Study the drawing (mm; zero at the part's minimum x, y, z) and answer. A direction names the side the tool comes from. Round coordinates to 2 decimals unless told otherwise and drop trailing zeros. Loops run counter-clockwise (first coordinate to the right, second up) from the corner with the lowest first, then second, coordinate; pieces in that order, holes last. Notation, with made-up numbers: (16, 9) - (72, 9) arc R20 ccw to (72, 36) - close; hole circle Ø10 at (23.25, 67.5). An arc over 180 degrees is marked (long way). Use CSV: the item, a comma, the result in double quotes. Start each with the question number.
1. Find section C-C (y = 16.5). Give the vertices of the cut face in (x, z), and give its area (3 significant figures).
2. Find section B-B (x = 5). Give the vertices of the cut face in (y, z), and give its area (3 significant figures).
3. Given pin 1 Ø4 at (x, z) = (17.73, 4) entering from -Y; pin 2 Ø2.5 at (x, z) = (17.73, 11.5) entering from -Y; pin 3 Ø3 at (y, z) = (18.5, 8.5) entering from +X; pin 4 Ø2 at (y, z) = (22, 2.5) entering from -X, each flat-ended and moving along its own axis, determine where each tip first touches the part or whether it passes through.
4. Find section A-A (y = 5). Give the vertices of the cut face in (x, z).
5. Determine the mould class of the marked faces 5, 6, 7 and 8 for opening direction X: +X half, -X half, draft (parallel to the pull), parting line (faces both ways), or undercut.
6. A tool of negligible diameter and unlimited length cuts with its end or side. For the marked faces 1, 2, 3 and 4, from which of +Z, -Z, +X, -X, +Y, -Y can it reach the whole face along a straight path? Write none if from no direction.
7. Consider line 1 along Y through (x, z) = (5, 4.75); line 2 along X through (y, z) = (32, 12.25) (1 decimal); line 3 along Y through (x, z) = (32.5, 6.25). Determine where each line is inside the solid, lowest interval first.
8. Find section D-D (z = 12.5). State how many separate pieces and enclosed holes the cut face has, and give its area (3 significant figures).
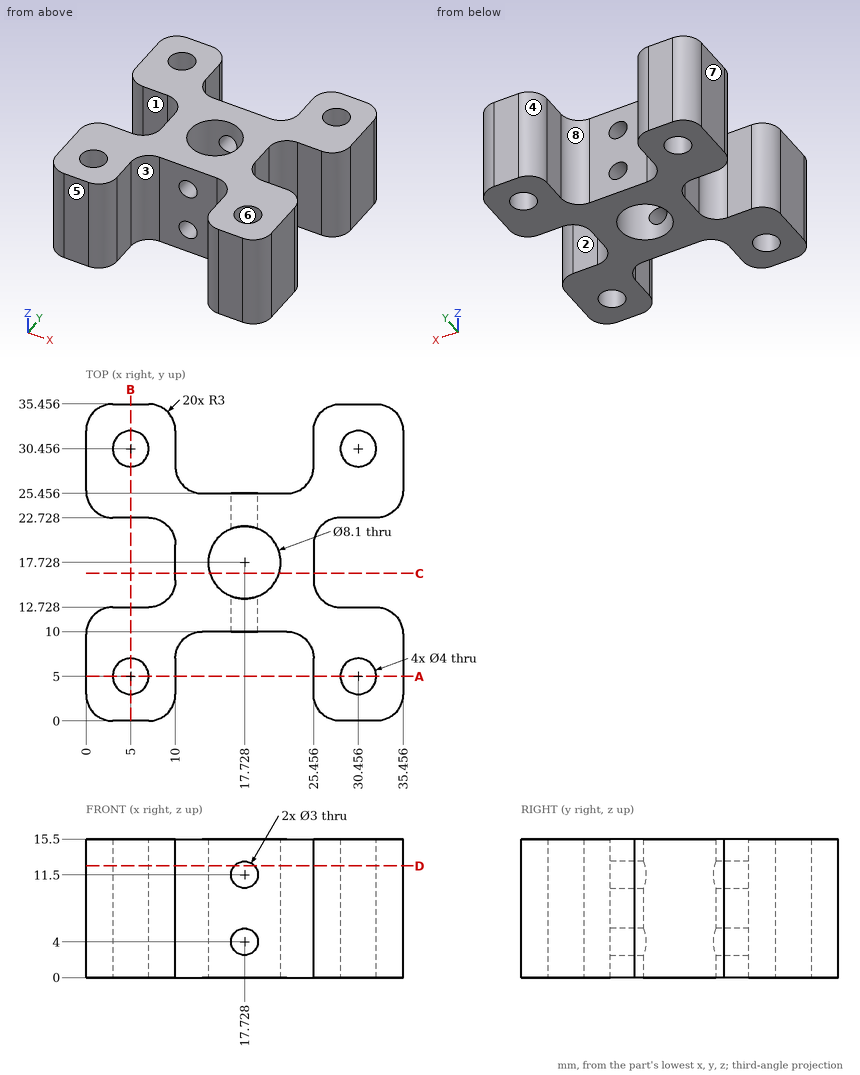
Filled sheet:
1,outline,"(10, 0) - (13.87, 0) - (13.87, 15.5) - (10, 15.5) - close; (21.59, 0) - (25.46, 0) - (25.46, 15.5) - (21.59, 15.5) - close"
1,area,"120 mm²"
2,outline,"(0, 0) - (3, 0) - (3, 15.5) - (0, 15.5) - close; (7, 0) - (12.73, 0) - (12.73, 15.5) - (7, 15.5) - close; (22.73, 0) - (28.46, 0) - (28.46, 15.5) - (22.73, 15.5) - close; (32.46, 0) - (35.46, 0) - (35.46, 15.5) - (32.46, 15.5) - close"
2,area,"271 mm²"
3,pin 1,"stops at y = 10"
3,pin 2,"passes through"
3,pin 3,"stops at x = 25.47"
3,pin 4,"stops at x = 1.75"
4,outline,"(0, 0) - (3, 0) - (3, 15.5) - (0, 15.5) - close; (7, 0) - (10, 0) - (10, 15.5) - (7, 15.5) - close; (25.46, 0) - (28.46, 0) - (28.46, 15.5) - (25.46, 15.5) - close; (32.46, 0) - (35.46, 0) - (35.46, 15.5) - (32.46, 15.5) - close"
5,face 5,"draft"
5,face 6,"undercut"
5,face 7,"-X half"
5,face 8,"undercut"
6,face 1,"+Z, -Z, -X"
6,face 2,"+Z, -Z, +X"
6,face 3,"+Z, -Z, -Y"
6,face 4,"+Z, -Z, +Y"
7,line 1,"y = 0 to 3, 7 to 12.73, 22.73 to 28.46, 32.46 to 35.46"
7,line 2,"x = 0 to 3.7, 6.3 to 10, 25.5 to 29.2, 31.7 to 35.5"
7,line 3,"y = 0 to 12.73, 22.73 to 35.46"
8,separate pieces,"2"
8,enclosed holes,"4"
8,area,"622 mm²"
